Here's how the part is built. I have some questions about the finished solid (model axes, mm). A direction names the side the tool comes from. Coordinates: 2 decimals unless noted, no trailing zeros. Loops run counter-clockwise (first coordinate to the right, second up) from the corner with the lowest first, then second, coordinate; pieces in that order, holes last.
Autodesk Fusion 360 part; units mm, degrees
sketch "Sketch1" plane through (0, 0, 0) normal (0, 1, 0) x (1, 0, 0)
  line L0 (32.5, 58) -> (-32.5, 58) construction
  line L1 (-32.5, 58) -> (-32.5, -58) construction
  line L2 (-32.5, -58) -> (32.5, -58) construction
  line L3 (32.5, -58) -> (32.5, 58) construction
  line L4 (32.5, 58) -> (-32.5, -58) construction
  line L5 (-32.5, 58) -> (32.5, -58) construction
  circle A0 centre (32.5, 58) radius 1.75
  line L6 (0, 0) -> (0, 14) construction
  line L7 (0, 0) -> (-15, 0) construction
  circle A1 centre (-32.5, 58) radius 1.75
  circle A2 centre (32.5, -58) radius 1.75
  circle A3 centre (-32.5, -58) radius 1.75
  line L8 (39.5, 65) -> (-39.5, 65)
  line L9 (-39.5, 65) -> (-39.5, -65)
  line L10 (-39.5, -65) -> (39.5, -65)
  line L11 (39.5, -65) -> (39.5, 65)
  line L12 (39.5, 65) -> (-39.5, -65) construction
  line L13 (-39.5, 65) -> (39.5, -65) construction
  line L14 (7.5, 85) -> (-7.5, 85)
  line L15 (-7.5, 85) -> (-7.5, 65)
  line L16 (-7.5, 65) -> (7.5, 65)
  line L17 (7.5, 65) -> (7.5, 85)
  line L18 (7.5, 85) -> (-7.5, 65) construction
  line L19 (-7.5, 85) -> (7.5, 65) construction
  circle A4 centre (0, 77) radius 3.25
  line L20 (-7.5, -85) -> (-7.5, -65)
  line L21 (7.5, -85) -> (-7.5, -85)
  line L22 (-7.5, -85) -> (7.5, -65) construction
  circle A5 centre (0, -77) radius 3.25
  line L23 (-7.5, -65) -> (7.5, -65)
  line L24 (7.5, -65) -> (7.5, -85)
  line L25 (7.5, -85) -> (-7.5, -65) construction
  point P0 (0, 75)
  point P1 (0, -75)
  dimension "d1" = 116
  dimension "d2" = 65
  dimension "d3" = 3.5
  dimension "d4" = 7
  dimension "d5" = 7
  dimension "d6" = 20
  dimension "d7" = 15
  dimension "d8" = 6.5
  dimension "d9" = 12
extrude "Extrude1" add sketch "Sketch1" along normal blind 4
fillet "Fillet1" radius 3 12 edges at (-39.5, 2, 65) (-7.5, 2, 85) (7.5, 2, 85) (7.5, 2, 65) (39.5, 2, 65) (39.5, 2, -65) (7.5, 2, -65) (7.5, 2, -85) (-7.5, 2, -85) (-39.5, 2, -65) (-7.5, 2, -65) (-7.5, 2, 65)
chamfer "Chamfer2" distance 2 angle 45 4 edges at (-34.1316, 4, 57.3672) (30.8684, 4, 57.3672) (30.8684, 4, -58.6328) (-34.1316, 4, -58.6328)
Q1. Suppose I cut it at A-A on y = 3.35. State how many separate pieces and enclosed holes the cut face has, and give its area (3 significant figures).
Q2. For faces 5 (the flat face through (7.5, 2, 75)), 6 (the flat face through (-1, 0, -1)), which set-ups out of +Z, -Z, +X, -X, +Y, -Y let a thin tool reach every point of the face, with its end or its side?
Q3. We'd pull the mould along X, two halves only. Please class faces 1 (the flat face through (-7.5, 2, -75)), 2 (the flat face through (24, 2, -65)), 3 (the cylindrical face through (-0.705, 1.972, -80.173)), 4 (the flat face through (7.5, 2, -75)): pulls with the +X half, pulls with the -X half, needs draft (parallel to the pull), parting line crosses it, or undercut.
Q4. Will these pins go through, and if not, where does the flat tip stop? P1, Ø2, axis at x = 29, y = 2, coming from the +Z side; P2, Ø2, axis at x = -6.5, y = 1.5, coming from the -Z side; P3, Ø2, axis at y = 2, z = -72, coming from the -X side.
Q5. Suppose I cut it at B-B on z = -77. Write out the boundary of the cut face in (x, y), and give its area (3 significant figures).
Q6. Please list where these lines run through material, in increasing order: probe 1 along Z at (x, y) = (0, 1.1); probe 2 along Z at (x, y) = (32.5, 1.15); probe 3 along X at (y, z) = (1.25, 58).
Q7. Suppose I cut it at D-D on z = -58. Write out the boundary of the cut face in (x, y).
Q8. Suppose I cut it at C-C on x = -32.5. Write out the boundary of the cut face in (y, z), and give its area (3 significant figures).
Check values:
1. separate pieces: 1
1. enclosed holes: 6
1. area: 10,700 mm2
2. face 5: +Z, +X, +Y, -Y
2. face 6: +Z, -Z, +X, -X, -Y
3. face 1: pulls with the -X half
3. face 2: needs draft
3. face 3: undercut
3. face 4: pulls with the +X half
4. P1: stops at z = 65
4. P2: stops at z = -84.83
4. P3: stops at x = -7.5
5. outline: (-7.5, 0) - (-3.25, 0) - (-3.25, 4) - (-7.5, 4) - close; (3.25, 0) - (7.5, 0) - (7.5, 4) - (3.25, 4) - close
5. area: 34.0 mm2
6. probe 1: z = -85 to -80.25, -73.75 to 73.75, 80.25 to 85
6. probe 2: z = -65 to -59.75, -56.25 to 56.25, 59.75 to 65
6. probe 3: x = -39.5 to -34.25, -30.75 to 30.75, 34.25 to 39.5
7. outline: (-39.5, 0) - (-34.25, 0) - (-34.25, 2) - (-36.25, 4) - (-39.5, 4) - close; (-30.75, 0) - (30.75, 0) - (30.75, 2) - (28.75, 4) - (-28.75, 4) - (-30.75, 2) - close; (34.25, 0) - (39.5, 0) - (39.5, 4) - (36.25, 4) - (34.25, 2) - close
8. outline: (0, -65) - (4, -65) - (4, -61.75) - (2, -59.75) - (0, -59.75) - close; (0, -56.25) - (2, -56.25) - (4, -54.25) - (4, 54.25) - (2, 56.25) - (0, 56.25) - close; (0, 59.75) - (2, 59.75) - (4, 61.75) - (4, 65) - (0, 65) - close
8. area: 484 mm2
